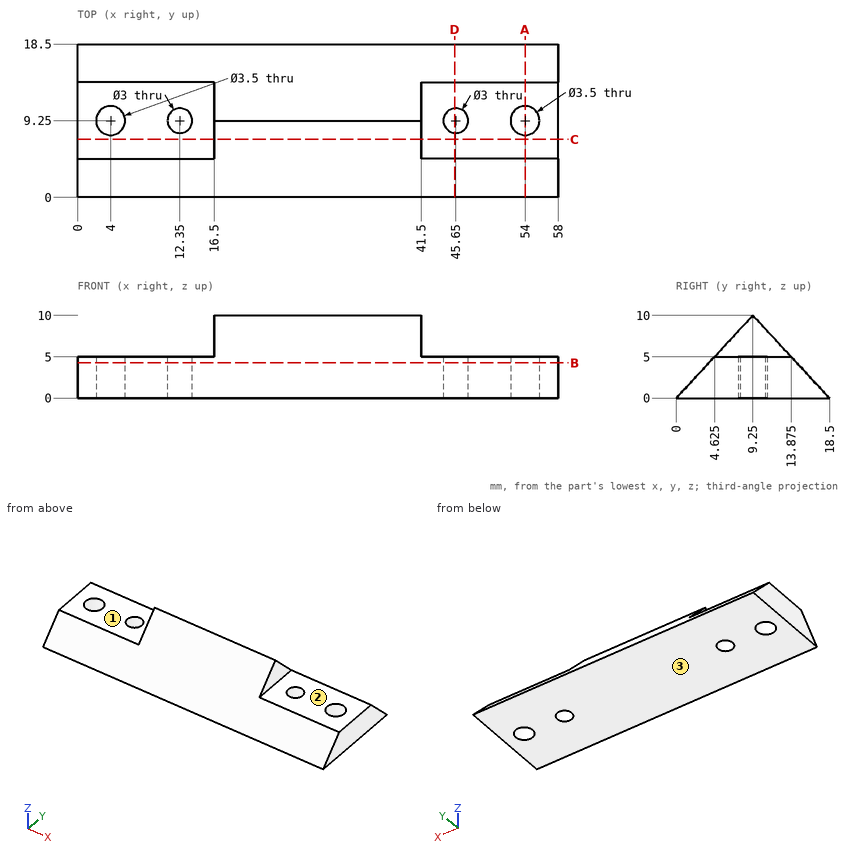
Drawing for the job (mm, zero at the part's lowest x, y, z). A direction names the side the tool comes from. Coordinates: 2 decimals unless noted, no trailing zeros. Order: outer loops, then holes, each group sorted by start corner. A loop starts at its lowest first (then second) coordinate and runs counter-clockwise, first axis right, second up.
Item 1: Band-saw the part on B-B on z = 4.25. List the corners of the cut face in (x, y), plus the area to 3 significant figures.
Check sheet entries:
outline: (0, 3.93) - (58, 3.93) - (58, 14.57) - (0, 14.57) - close; hole circle Ø3.5 at (4, 9.25); hole circle Ø3 at (12.35, 9.25); hole circle Ø3 at (45.65, 9.25); hole circle Ø3.5 at (54, 9.25)
area: 584 mm2
Item 2: Drill centre lines: L1, parallel to X at y = 10.5, z = 3.5; L2, parallel to X at y = 10, z = 7; L3, parallel to Y at x = 12.35, z = 1.85. Where is each one in solid material? Low to high.
Check sheet entries:
L1: x = 0 to 2.78, 5.22 to 11.52, 13.18 to 44.82, 46.48 to 52.78, 55.22 to 58
L2: x = 16.5 to 41.5
L3: y = 1.71 to 7.75, 10.75 to 16.79
Item 3: Band-saw the part on D-D on x = 45.5. List the corners of the cut face in (y, z) (3 decimals), plus the area to 3 significant figures.
Check sheet entries:
outline: (0, 0) - (7.758, 0) - (7.758, 5) - (4.625, 5) - close; (10.742, 0) - (18.5, 0) - (13.875, 5) - (10.742, 5) - close
area: 54.5 mm2
Item 4: Band-saw the part on C-C on y = 7. List the corners of the cut face in (x, z), plus the area to 3 significant figures.
Check sheet entries:
outline: (0, 0) - (58, 0) - (58, 5) - (41.5, 5) - (41.5, 7.57) - (16.5, 7.57) - (16.5, 5) - (0, 5) - close
area: 354 mm2
Item 5: 3-axis set-ups, long thin cutter, end or side, ignore diameter. For the marked faces 1, 2 and 3: which of +Z, -Z, +X, -X, +Y, -Y reach the whole face in a straight line?
Check sheet entries:
face 1: +Z, -X, +Y, -Y
face 2: +Z, +X, +Y, -Y
face 3: -Z, +X, -X, +Y, -Y
Item 6: Band-saw the part on A-A on x = 54. List the corners of the cut face in (y, z) (3 decimals), plus the area to 3 significant figures.
Check sheet entries:
outline: (0, 0) - (7.5, 0) - (7.5, 5) - (4.625, 5) - close; (11, 0) - (18.5, 0) - (13.875, 5) - (11, 5) - close
area: 51.9 mm2
Item 7: Pin check, flat tips, straight feed: pin 1 Ø2 at (x, y) = (54, 9.25) entering from -Z; pin 2 Ø3 at (x, y) = (5, 9.5) entering from +Z; pin 3 Ø3 at (x, z) = (24.5, 7.5) entering from -Y; pin 4 Ø4 at (x, z) = (40.5, 6) entering from -Y. Stop position of each tip, or through.
Check sheet entries:
pin 1: passes through
pin 2: stops at z = 5
pin 3: stops at y = 5.55
pin 4: stops at y = 3.7
